Part model, mm, in its own coordinate system. A direction names the side the tool comes from. Coordinates: 2 decimals unless noted, no trailing zeros. Write each loop counter-clockwise with the first axis right and the second up, starting at its lowest first coordinate (ties: lowest second). Pieces come first, ordered by that corner, then holes. Notation, with made-up numbers: M 58,81.25 L 111,81.25 A7 cw 111,92.25 Z; hole C -39.75,-28 d7. An arc over 180 degrees is marked long. Use a Markdown table: item, result. Add a question column.
Q1. Slice it at C-C on z = 306.5. Write the cut outline in (x, y), then the cut area to 3 significant figures.
Q2. Tool access for faces 1 (the flat face through (3, 15, 380)), 2 (the flat face through (0, -35, -25)): list every direction of +Z, -Z, +X, -X, +Y, -Y with a clear straight run to the whole face (end or side of a thin tool).
Q3. Slice it at A-A on x = 0. Write the cut outline in (y, z), then the cut area to 3 significant figures.
Q4. Pin check, flat tips, straight feed: pin 1 Ø12 at (x, z) = (-24.5, 28.5) entering from +Y; pin 2 Ø1 at (y, z) = (-3, 288) entering from -X; pin 3 Ø10 at (x, z) = (-13.5, 140) entering from -Y; pin 4 Ø5 at (x, z) = (23, 45.5) entering from -Y. Stop position of each tip, or through.
Q5. Slice it at D-D on y = -28.5. Write the cut outline in (x, z).
Q6. Wall check: L1, parallel to Z at x = -20, y = -12; L2, parallel to Z at x = 10.5, y = -16.5; L3, parallel to Y at x = 9.5, z = 184.5. Give the ranges that are in metal, low to high. Write a range as from..to.
from build123d import *

# Parameters (mm, degrees)
SKETCH2_R           = 20
BOSS_EXTRUDE2_DEPTH = 380
SKETCH4_W           = 70
SKETCH4_H           = 70
BOSS_EXTRUDE3_DEPTH = 50
SKETCH5_R           = 15
BOSS_EXTRUDE4_DEPTH = 20


with BuildPart() as part:
    # Sketch2 → Boss-Extrude2 (new body)
    with BuildSketch(Plane.XY):
        Circle(SKETCH2_R)
    extrude(amount=BOSS_EXTRUDE2_DEPTH)

    # Sketch4 → Boss-Extrude3 (add)
    with BuildSketch(Plane(origin=(0, 0, 0), x_dir=(-1, 0, 0), z_dir=(0, 0, -1))):
        Rectangle(SKETCH4_W, SKETCH4_H)
    extrude(amount=BOSS_EXTRUDE3_DEPTH)

    # Sketch5 → Boss-Extrude4 (add)
    with BuildSketch(Plane.XY.offset(380)):
        Circle(SKETCH5_R)
    extrude(amount=BOSS_EXTRUDE4_DEPTH)


solid = part.part
Recorded:
| question | item | result |
|---|---|---|
| 1 | outline | C 0,0 d40 |
| 1 | area | 1,260 mm² |
| 2 | face 1 | +Z |
| 2 | face 2 | +Z, -Z, +X, -X, -Y |
| 3 | outline | M -35,-50 L 35,-50 L 35,0 L 20,0 L 20,380 L 15,380 L 15,400 L -15,400 L -15,380 L -20,380 L -20,0 L -35,0 Z |
| 3 | area | 19,300 mm² |
| 4 | pin 1 | y = 7.6 |
| 4 | pin 2 | x = -19.84 |
| 4 | pin 3 | y = -18.1 |
| 4 | pin 4 | through |
| 5 | outline | M -35,-50 L 35,-50 L 35,0 L -35,0 Z |
| 6 | L1 | -50..0 |
| 6 | L2 | -50..380 |
| 6 | L3 | -17.6..17.6 |
